Solid Edge part; units mm, degrees
sketch "Sketch1" plane through (0, 0, 25) normal (0, 0, 1) x (1, 0, 0)
  line L0 (-49.5, -36.5) -> (-19.5, -36.5)
  line L1 (-19.5, 6.5) -> (-19.5, -36.5)
  line L2 (-19.5, 6.5) -> (-49.5, 6.5)
  line L3 (-49.5, 6.5) -> (-49.5, -36.5)
  circle A0 centre (-25, -31) radius 2.2
  circle A1 centre (-44, 1) radius 2.2
  circle A2 centre (-25, 1) radius 2.2
  circle A3 centre (-44, -31) radius 2.2
extrude "ExtrudedProtrusion_1" add sketch "Sketch1" along normal blind 15
sketch "Sketch2" plane through (-34.5, -36.5, 32.5) normal (0, -1, 0) x (0, 0, 1)
  circle A0 centre (-7.5, 0) radius 4
extrude "Cutout1" cut sketch "Sketch2" against normal through all
sketch "Sketch3" plane through (-34.5, -36.5, 32.5) normal (0, -1, 0) x (1, 0, 0)
  line L0 (-5, 7.5) -> (-5, 1.5)
  line L1 (-5, 1.5) -> (5, 1.5)
  line L2 (5, 7.5) -> (5, 1.5)
extrude "Cutout2" cut sketch "Sketch3" against normal through all material side at (-39.45, -36.5, 37)
sketch "Sketch4" plane through (-24.5, -15, 40) normal (0, 0, 1) x (0, 1, 0)
  line L0 (-10.5, 25) -> (-10.5, 12.5)
extrude "Cutout3" cut sketch "Sketch4" against normal through all material side at (-43.25, -25.45, 40)
fillet "Round_1" radius 1 2 edges at (-39.5, -31, 34) (-29.5, -31, 34)
sketch "Sketch5" plane through (-44.5, -31, 40) normal (0, 0, 1) x (1, 0, 0)
  line L0 (0.5, 0) -> (2.0825, 1.5282)
  line L1 (2.0825, 1.5282) -> (0.5, 3.167)
  line L2 (0.5, 3.167) -> (-1.0825, 1.5282)
  line L3 (-1.0825, 1.5282) -> (0.5, 0)
  line L4 (19.5, 0) -> (21.0825, 1.5282)
  line L5 (21.0825, 1.5282) -> (19.5, 3.167)
  line L6 (19.5, 3.167) -> (17.9175, 1.5282)
  line L7 (17.9175, 1.5282) -> (19.5, 0)
extrude "Cutout4" cut sketch "Sketch5" against normal through all
Read the model definition and answer for the solid it produces. Units are mm, in the model's axes. A direction names the side the tool comes from. Give positions to 0.01 mm unless a question says otherwise; leave off trailing zeros. Write each loop counter-clockwise with the first axis right and the second up, starting at its lowest first coordinate (ties: lowest second). Pieces come first, ordered by that corner, then holes. Notation, with made-up numbers: (66.25, 58) -> (121.25, 58) arc R11 cw to (121.25, 73) -> close; hole circle Ø1 at (-36.5, 69). An arc over 180 degrees is marked (long way). Answer as a JSON object with one key per item and string values. Group by question number.
1) Find section A-A (z = 37.25). Write down the section's boundary in (x, y).
2) Find section D-D (y = -27.25). Write down the section's boundary in (x, z).
3) A tool of negligible diameter and unlimited length cuts with its end or side. For faces 5 (the flat face through (-29.5, -31, 38)), 6 (the cylindrical face through (-34.4, -31.1, 29)), 7 (the flat face through (-25.77, -28.63, 32.61)), from which of +Z, -Z, +X, -X, +Y, -Y can it reach the whole face along a straight path? Write none if from no direction.
4) Find section B-B (z = 29.75). Write down the section's boundary in (x, y).
5) Find section C-C (y = -31). Write down the section's boundary in (x, z), and give its area (3 significant figures).
6) This flat-tipped pin is pushed along its axis until it touches: P1, Ø1, axis at x = -38.5, y = -29, coming from the +Z side. Where does it stop, or does it pass through?
7) The mould has two halves that part along X. Classify faces 1 (the flat face through (-19.5, -31, 32)), 2 (the cylindrical face through (-29.785, -30.923, 34.301)), 3 (the cylindrical face through (-43.93, -33.2, 32.39)), 4 (the flat face through (-35, -25.5, 33)): +X half, -X half, draft (parallel to the pull), parting line (faces both ways), or undercut.
8) Consider L1, parallel to X at y = -31, z = 32.5; L2, parallel to X at y = -31, z = 35.75; L3, parallel to X at y = -28, z = 36. Determine where each line is inside the solid, lowest interval first. Write a range as from..to.
Values follow:
{
 "1": {"outline": "(-49.5, -36.5) -> (-39.5, -36.5) -> (-39.5, -25.5) -> (-49.5, -25.5) -> close; (-29.5, -36.5) -> (-19.5, -36.5) -> (-19.5, -25.5) -> (-29.5, -25.5) -> close; hole (-45.57, -29.46) arc R2.2 ccw (long way) to (-42.43, -29.46) -> (-44, -27.83) -> close; hole (-26.57, -29.46) arc R2.2 ccw (long way) to (-23.43, -29.46) -> (-25, -27.83) -> close"},
 "2": {"outline": "(-49.5, 25) -> (-38.5, 25) arc R4 cw to (-30.5, 25) -> (-19.5, 25) -> (-19.5, 40) -> (-29.5, 40) -> (-29.5, 35) arc R1 cw to (-30.5, 34) -> (-38.5, 34) arc R1 cw to (-39.5, 35) -> (-39.5, 40) -> (-49.5, 40) -> close"},
 "3": {"face 5": "+Z, +Y, -Y", "face 6": "-Z, +Y, -Y", "face 7": "+Z, -Z"},
 "4": {"outline": "(-49.5, -36.5) -> (-19.5, -36.5) -> (-19.5, -25.5) -> (-49.5, -25.5) -> close; hole (-45.57, -29.46) arc R2.2 ccw (long way) to (-42.43, -29.46) -> (-44, -27.83) -> close; hole (-26.57, -29.46) arc R2.2 ccw (long way) to (-23.43, -29.46) -> (-25, -27.83) -> close"},
 "5": {"outline": "(-49.5, 25) -> (-46.2, 25) -> (-46.2, 40) -> (-49.5, 40) -> close; (-41.8, 25) -> (-38.5, 25) arc R4 cw to (-30.5, 25) -> (-27.2, 25) -> (-27.2, 40) -> (-29.5, 40) -> (-29.5, 35) arc R1 cw to (-30.5, 34) -> (-38.5, 34) arc R1 cw to (-39.5, 35) -> (-39.5, 40) -> (-41.8, 40) -> close; (-22.8, 25) -> (-19.5, 25) -> (-19.5, 40) -> (-22.8, 40) -> close", "area": "233 mm2"},
 "6": {"P1": "stops at z = 34.13"},
 "7": {"face 1": "+X half", "face 2": "undercut", "face 3": "undercut", "face 4": "draft"},
 "8": {"L1": "x = -49.5..-46.2, -41.8..-27.2, -22.8..-19.5", "L2": "x = -49.5..-46.2, -41.8..-39.5, -29.5..-27.2, -22.8..-19.5", "L3": "x = -49.5..-44.16, -43.84..-39.5, -29.5..-25.16, -24.84..-19.5"}
}
